```python
from build123d import *

# Parameters (mm, degrees)
F3_R     = 0.25
F4_SIZE2 = 0.1763269807
F4_SIZE  = 1
F6_D     = 3
F6_DEPTH = 3
F6_TIP   = 0.9012909285


# Not quite as in the source:
# - a fillet or chamfer that OpenCascade refuses, or shapes differently, is made with other operations: its cross-section is extruded or revolved along the edge and cut away or added


with BuildPart() as f1:
    # F0 (on Right) → F1 (revolve)
    with BuildSketch(Plane.YZ):
        Polygon((0, 0), (-4.75, 0), (-4.75, -4.5), (-2.5, -4.5), (-2.5, -8), (0, -8), align=None)
    revolve(axis=Axis((0, 0, -4), (0, 0, -1)))

    # F2: chamfer of 0.5 x 0.1819851171 on 1 edges, made by hand

    # F2_s1 → F2_t2 (revolve, cut)
    with BuildSketch(Plane.YZ):
        Polygon((-4.5680148829, 0), (-4.75, -0.5), (-4.75, 0), align=None)
    revolve(axis=Axis((0, 0, 0), (0, 0, -1)), mode=Mode.SUBTRACT)

    # F3
    f3_edges = [f1.edges().sort_by_distance(p)[0] for p in [
        (0, 4.75, -4.5),
        (0, 2.5, -4.5),
    ]]
    fillet(f3_edges, radius=F3_R)

    # F4
    f4_edges = [f1.edges().sort_by_distance(p)[0] for p in [
        (0, 2.5, -8),
    ]]
    chamfer(f4_edges, length=F4_SIZE, length2=F4_SIZE2)

    # F6
    with Locations(Plane(origin=(0, 0, -8), x_dir=(1, 0, 0), z_dir=(0, 0, -1))):
        with Locations((0, 0)):
            Hole(F6_D / 2, depth=F6_DEPTH)
            with Locations((0, 0, -(F6_DEPTH + F6_TIP / 2))):  # 118° drill point
                Cone(0, F6_D / 2, F6_TIP, mode=Mode.SUBTRACT)


solid = f1.part
```
Work out the finished part from the listing and answer in its coordinate system (mm). A direction names the side the tool comes from. Round coordinates to 2 decimals unless told otherwise and drop trailing zeros. Loops run counter-clockwise (first coordinate to the right, second up) from the corner with the lowest first, then second, coordinate; pieces in that order, holes last. Notation, with made-up numbers: (31, -40) -> (37, -40) arc R12 ccw to (37, -21) -> close; hole circle Ø5 at (65.25, -27.75). An arc over 180 degrees is marked (long way). Write each question's results on one line, items separated by ' | '. Start each with the question number.
1. Section A-A (z = -6.75) is taken. Determine the outline of the cut face in (x, y).
2. For a pull along Y with two mould halves and no side action, classify faces 1 (the face through (1.5, -0.07, -6.48)), 2 (the face through (3, 0, -4.5)), 3 (the face through (4.214, -2.192, -2.401)) as +Y half, -Y half, draft (parallel to the pull), parting line (faces both ways), or undercut.
3. A tool of negligible diameter and unlimited length cuts with its end or side. For faces 4 (the face through (0, 0, 0)), 5 (the face through (2.44, 0.54, -5.89)), from which of +Z, -Z, +X, -X, +Y, -Y can it reach the whole face along a straight path? Write none if from no direction.
4. Section B-B (z = -1.75) is taken. Determine the outline of the cut face in (x, y).
5. Find the intervals of material crossed by probe 1 along Y at (x, z) = (0, -6.2); probe 2 along Z at (x, y) = (-2.5, 2.5); probe 3 along Y at (x, z) = (-1, -6.25), in increasing order. Write a range as from..to.
6. Given pin 1 Ø2 at (y, z) = (-2, -4) entering from +X; pin 2 Ø2.5 at (x, y) = (0, 0) entering from -Z; pin 3 Ø3 at (y, z) = (1, -1.5) entering from -X, each flat-ended and moving along its own axis, determine where each tip first touches the part or whether it passes through.
Evaluation:
1) outline: circle Ø5 at (0, 0); hole circle Ø3 at (0, 0)
2) face 1: undercut | face 2: draft | face 3: parting line
3) face 4: +Z, +X, -X, +Y, -Y | face 5: -Z
4) outline: circle Ø9.5 at (0, 0)
5) probe 1: y = -2.5..-1.5, 1.5..2.5 | probe 2: z = -4.5..0 | probe 3: y = -2.29..-1.12, 1.12..2.29
6) pin 1: stops at x = 4.64 | pin 2: stops at z = -4.85 | pin 3: stops at x = -4.75
